The model under review builds one solid part; all positions refer to its coordinate system, in mm. Face numbers are marked on the shaded views. Coordinates: 2 decimals unless noted, no trailing zeros. Write each question's results on one line, items separated by ' | '.
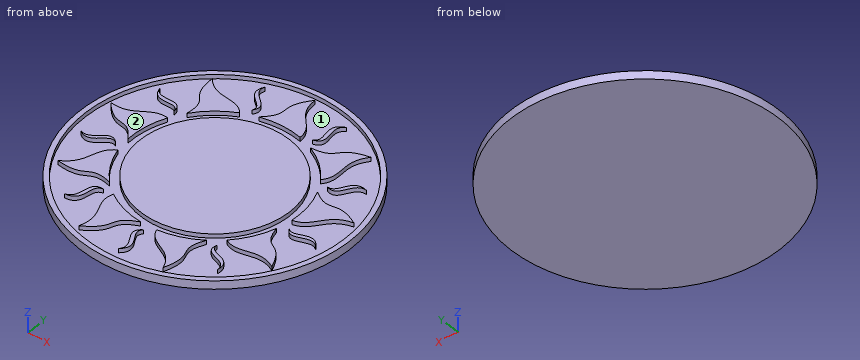
from build123d import *

# Parameters (mm, degrees)
F0_R     = 32.5
F1_DEPTH = 2
F2_R     = 31.3
F2_R_2   = 18
F3_DEPTH = 1
F5_DEPTH = 1
F6_COUNT = 9


with BuildPart() as f1:
    # F0 (on Top) → F1 (new body)
    with BuildSketch(Plane.XY):
        Circle(F0_R)
    extrude(amount=F1_DEPTH)

    # F2 (on face) → F3 (cut)
    with BuildSketch(Plane.XY.offset(2)):
        Circle(F2_R)
        Circle(F2_R_2, mode=Mode.SUBTRACT)
    extrude(amount=-F3_DEPTH, mode=Mode.SUBTRACT)

    # F4 (on face) → F5 (join, through all)
    with BuildSketch(Plane.XY.offset(1)):
        with BuildLine():
            ThreePointArc((-5, 19.364916731), (0, 20), (5, 19.364916731))
            add(Edge.make_bspline(
                [(0, 30), (0, 24), (5, 24), (5, 19.364916731)],
                knots=[0, 0, 0, 0, 11.7518082072, 11.7518082072, 11.7518082072, 11.7518082072], degree=3))
            add(Edge.make_bspline(
                [(-5, 19.364916731), (0, 24), (-5, 24), (0, 30)],
                knots=[0, 0, 0, 0, 11.7518082072, 11.7518082072, 11.7518082072, 11.7518082072], degree=3))
        make_face()
        with BuildLine():
            add(Edge.make_bspline(
                [(9.9131672787, 27.2362032534), (6.7328927107, 25.4915188998), (11.3224480301, 21.147036925), (7.3497492192, 20.1932700184)],
                knots=[0, 0, 0, 0, 7.4949330017, 7.4949330017, 7.4949330017, 7.4949330017], degree=3))
            add(Edge.make_bspline(
                [(9.9131672787, 27.2362032534), (5.5151497945, 25.5608577281), (10.0525226444, 21.4589480311), (7.3497492192, 20.1932700184)],
                knots=[0, 0, 0, 0, 7.4949330017, 7.4949330017, 7.4949330017, 7.4949330017], degree=3))
        make_face()
    extrude(amount=F5_DEPTH)

    # F6: F1 ×9 about axis
    f6_axis = Axis((0, 0, 0), (0, 0, -1))


with BuildPart() as f1_1:
    add(f1.part)
    for i in range(1, F6_COUNT):
        add(f1.part.rotate(f6_axis, i * 360 / F6_COUNT))


solid = f1_1.part
1) The part is to be moulded in two halves that separate along Y. For the marked faces 1 and 2, say which applies: pulls with the +Y half, pulls with the -Y half, needs draft (parallel to the pull), parting line crosses it, or undercut.
Solutions:
face 1: undercut | face 2: needs draft
2) To check wall thickness, follow line 1 along Y through (x, z) = (16, 1.75); line 2 along X through (y, z) = (0, 1.7); line 3 along Z through (x, y) = (-9, 29). State the ranges of each line that lie inside material, in increasing order.
Solutions:
line 1: -28.29 to -26.9, -19.51 to -18.56, -14.66 to -12, -8.25 to 8.25, 12 to 22.03, 26.9 to 28.29 | line 2: -32.5 to -31.3, -21.09 to -20, -18 to 18, 20 to 22.85, 31.3 to 32.5 | line 3: 0 to 1
3) Take a section at A-A on z = 1.65. Count the separate pieces of the cut face and the enclosed holes in it, plus the area to 3 significant figures.
Solutions:
separate pieces: 20 | enclosed holes: 1 | area: 1,710 mm2
4) For pin 1 (1 mm diameter, centred on x = 15.5, z = 0.5, fed in from +Y), flat-tipped, find the tip position at first contact; note if it passes through.
Solutions:
pin 1: y = 28.83
